```python
from build123d import *

# Parameters (mm, degrees)
SKETCH2_W               = 266.7
SKETCH2_H               = 1016
BOSS_EXTRUDE1_DEPTH     = 6.35
CAVITY1_START           = -6.35
CAVITY1_OUTLINE_R       = 12.7
CAVITY1_DEPTH           = 12.7
CAVITY1_START_2         = 449.025238005
CAVITY1_2_OUTLINE_R     = 12.7
CAVITY1_2_DEPTH         = 39.100356678
CUT_EXTRUDE3_DEPTH      = 1025.733401915
CUT_EXTRUDE3_DEPTH_BACK = 1025.733401915
SKETCH5_W               = 12.7
SKETCH5_H               = 508


# Read off the part's stored shape, not the designer's step: Cavity1
with BuildPart() as part:
    # Sketch2 → Boss-Extrude1 (new, symmetric)
    with BuildSketch(Plane.XY):
        with Locations((0, 508)):
            Rectangle(SKETCH2_W, SKETCH2_H)
    extrude(amount=BOSS_EXTRUDE1_DEPTH, both=True)

    # Cavity1 outline → Cavity1 (cut)
    with BuildSketch(Plane.XY.offset(CAVITY1_START)):
        with Locations((-69.85, 819.9)):
            Circle(CAVITY1_OUTLINE_R)
        with Locations((-69.85, 469.9)):
            Circle(CAVITY1_OUTLINE_R)
    extrude(amount=CAVITY1_DEPTH, mode=Mode.SUBTRACT)

    # Cavity1 2 outline → Cavity1 2 (cut)
    with BuildSketch(Plane(origin=(0, 0, 0), x_dir=(1, 0, 0), z_dir=(0, 0.658504607868519, 0.752576694706877)).offset(CAVITY1_START_2)):
        with Locations((-69.85, 535.514761536)):
            Circle(CAVITY1_2_OUTLINE_R)
    extrude(amount=CAVITY1_2_DEPTH, mode=Mode.SUBTRACT)

    # Sketch5 → Cut-Extrude3 (cut, two sides: drawn at the far end of the back side and taken through both)
    with BuildSketch(Plane.XY.offset(-CUT_EXTRUDE3_DEPTH_BACK)):
        with Locations((63.5, 762)):
            Rectangle(SKETCH5_W, SKETCH5_H)
    extrude(amount=CUT_EXTRUDE3_DEPTH + CUT_EXTRUDE3_DEPTH_BACK, mode=Mode.SUBTRACT)


solid = part.part
```
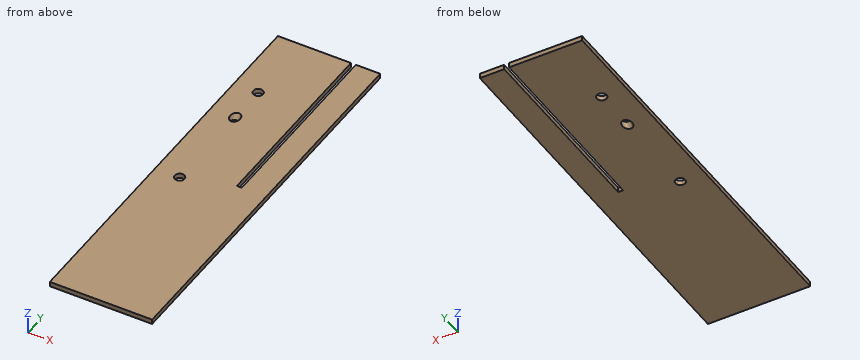
Source: CAD feature listing. Evaluate the final solid. Frame: model axes, mm. Round coordinates to 2 decimals unless told otherwise and drop trailing zeros. Loops run counter-clockwise (first coordinate to the right, second up) from the corner with the lowest first, then second, coordinate; pieces in that order, holes last.
1. Section query C-C on x = -69.85. Output: boundary loops of the cut face in (y, z), and give its area (3 significant figures).
2. Section query B-B on y = 819.9. Output: boundary loops of the cut face in (x, z), and give its area (3 significant figures).
3. Ray query, L1, parallel to X at y = 582, z = 2.5; L2, parallel to X at y = 819.9, z = -1.5; L3, parallel to Y at x = -69.85, z = 1.25. Return the intervals inside material, ascending.
4. Section query A-A on y = 469.9. Output: boundary loops of the cut face in (x, z).
5. Section query D-D on y = 669. Output: boundary loops of the cut face in (x, z), and give its area (3 significant figures).
6. Contact query for a flat-ended pin moving along its axis: pin 1 (1.5 mm diameter, centred on x = -50, z = -1.5, fed in from -Y). Output: stop coordinate, or through.
Answers below:
1. outline: (0, -6.35) - (457.2, -6.35) - (457.2, 6.35) - (0, 6.35) - close; (482.6, -6.35) - (689.14, -6.35) - (700.26, 6.35) - (482.6, 6.35) - close; (722.89, -6.35) - (807.2, -6.35) - (807.2, 6.35) - (734.01, 6.35) - close; (832.6, -6.35) - (1016, -6.35) - (1016, 6.35) - (832.6, 6.35) - close
1. area: 11,800 mm2
2. outline: (-133.35, -6.35) - (-82.55, -6.35) - (-82.55, 6.35) - (-133.35, 6.35) - close; (-57.15, -6.35) - (57.15, -6.35) - (57.15, 6.35) - (-57.15, 6.35) - close; (69.85, -6.35) - (133.35, -6.35) - (133.35, 6.35) - (69.85, 6.35) - close
2. area: 2,900 mm2
3. L1: x = -133.35 to 57.15, 69.85 to 133.35
3. L2: x = -133.35 to -82.55, -57.15 to 57.15, 69.85 to 133.35
3. L3: y = 0 to 457.2, 482.6 to 695.79, 729.54 to 807.2, 832.6 to 1016
4. outline: (-133.35, -6.35) - (-82.55, -6.35) - (-82.55, 6.35) - (-133.35, 6.35) - close; (-57.15, -6.35) - (133.35, -6.35) - (133.35, 6.35) - (-57.15, 6.35) - close
5. outline: (-133.35, -6.35) - (57.15, -6.35) - (57.15, 6.35) - (-133.35, 6.35) - close; (69.85, -6.35) - (133.35, -6.35) - (133.35, 6.35) - (69.85, 6.35) - close
5. area: 3,230 mm2
6. pin 1: stops at y = 0
